The figure shows three views and two pictorial views of one solid part (mm, origin at its lowest corner). Answer the questions. Coordinates: 2 decimals unless noted, no trailing zeros. Loops run counter-clockwise (first coordinate to the right, second up) from the corner with the lowest first, then second, coordinate; pieces in that order, holes last.
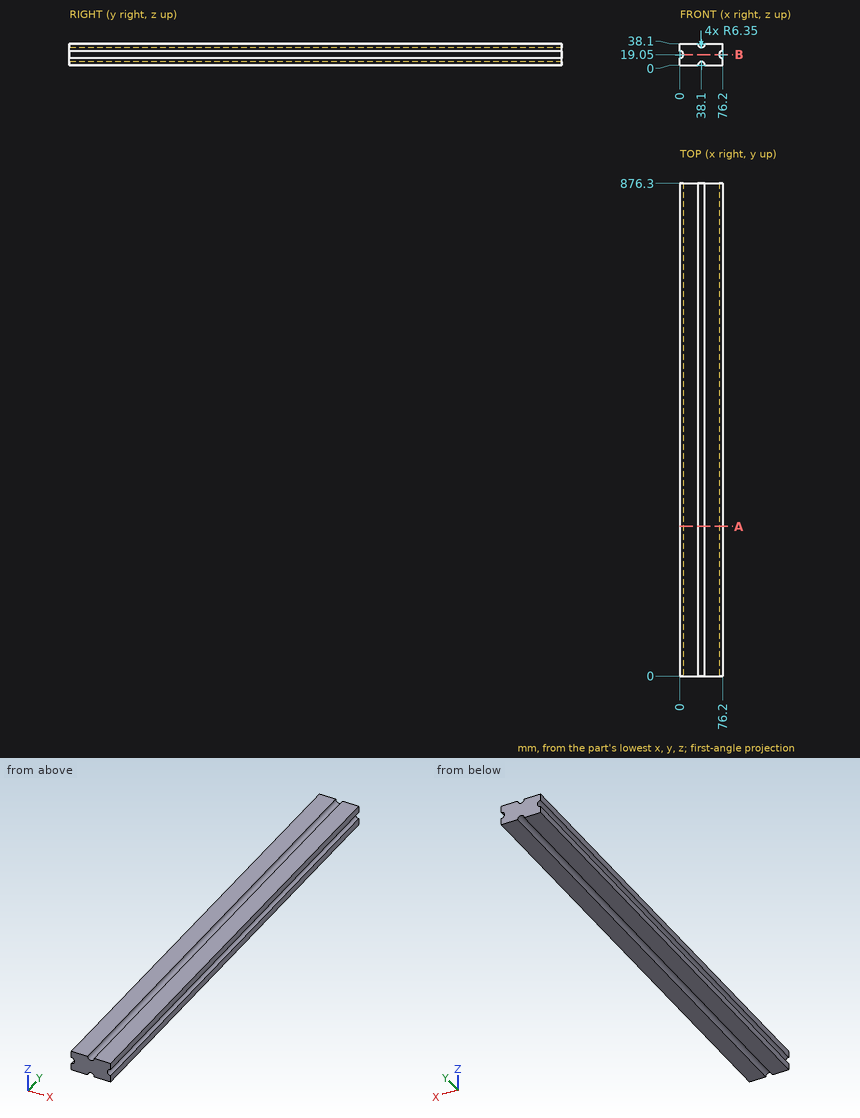
Q1. A cutting plane is placed at B-B (z = 19.05). Give the vertices of the cut face in (x, y), then the cut area to 3 significant figures.
Findings below:
outline: (6.35, 0) - (69.85, 0) - (69.85, 876.3) - (6.35, 876.3) - close
area: 55,600 mm2
Q2. Straight lines are drawn through the part: probe 1 along X at (y, z) = (533.5, 20); probe 2 along Z at (x, y) = (5.5, 812); probe 3 along X at (y, z) = (547.5, 5.5). For each, find the intervals that lie inside material, in ascending order.
Findings below:
probe 1: x = 6.28 to 69.92
probe 2: z = 0 to 15.88, 22.22 to 38.1
probe 3: x = 0 to 34.93, 41.27 to 76.2
Q3. Flat-ended cylindrical pins translate along their axes: pin 1 Ø3 at (x, y) = (32, 674) entering from -Z; pin 2 Ø1 at (y, z) = (389.5, 16.5) entering from +X; pin 3 Ø1.5 at (y, z) = (525.5, 17.5) entering from +X. Find the tip coordinate at first contact, or state that the pin passes through.
Findings below:
pin 1: stops at z = 0
pin 2: stops at x = 70.63
pin 3: stops at x = 70.28
Q4. A cutting plane is placed at A-A (y = 266). Give the vertices of the cut face in (x, z).
Findings below:
outline: (0, 0) - (31.75, 0) arc R6.35 cw to (44.45, 0) - (76.2, 0) - (76.2, 12.7) arc R6.35 cw to (76.2, 25.4) - (76.2, 38.1) - (44.45, 38.1) arc R6.35 cw to (31.75, 38.1) - (0, 38.1) - (0, 25.4) arc R6.35 cw to (0, 12.7) - close
